Drawing for the job (mm, zero at the part's lowest x, y, z). A direction names the side the tool comes from. Give positions to 0.01 mm unless a question says otherwise; leave off trailing zeros. Write each loop counter-clockwise with the first axis right and the second up, starting at its lowest first coordinate (ties: lowest second). Pieces come first, ordered by that corner, then holes. Notation, with made-up numbers: (-2, 44.25) - (8, 44.25) arc R32 ccw to (8, 79.25) - close; hole circle Ø10 at (3.25, 5.25). An arc over 180 degrees is marked (long way). Write item = value, one per line. Start each with the question number.
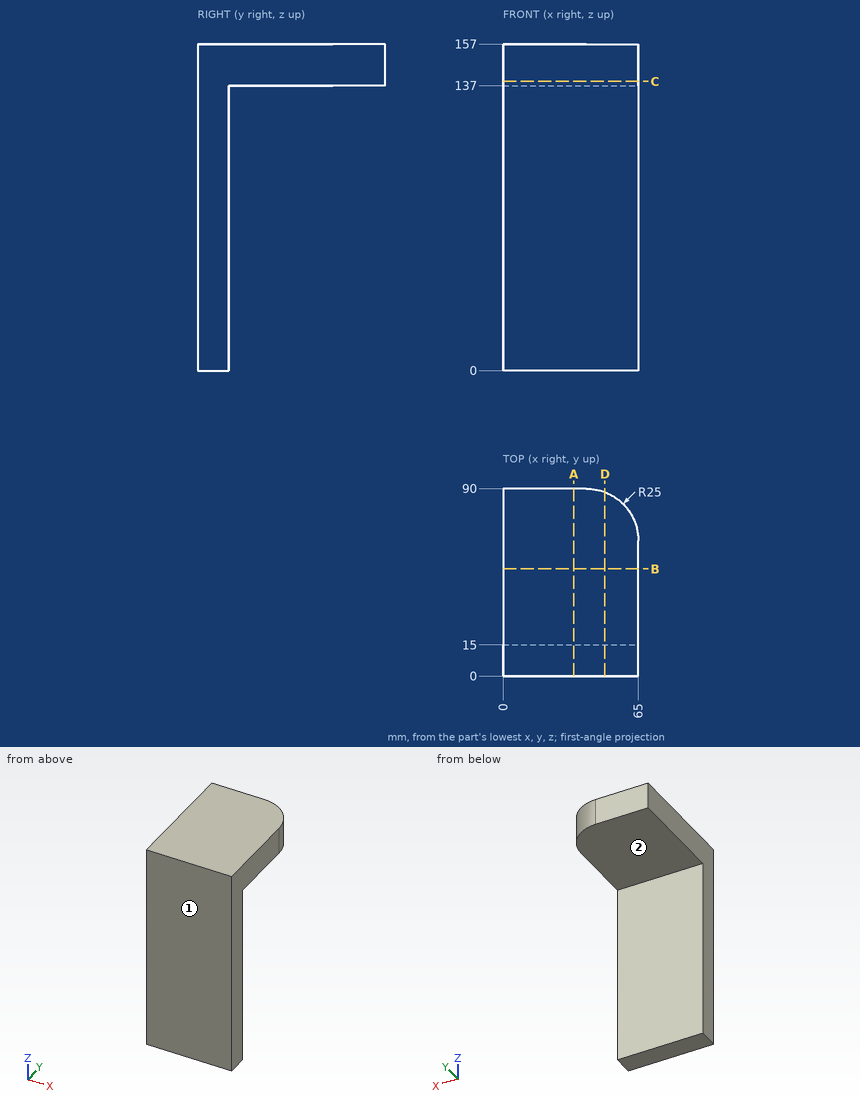
1. Tool access for the marked faces 1 and 2: list every direction of +Z, -Z, +X, -X, +Y, -Y with a clear straight run to the whole face (end or side of a thin tool).
2. Cut at C-C (z = 139). Give the cut face in (x, y).
3. Cut at A-A (x = 34). Give the cut face in (y, z).
4. Cut at B-B (y = 51.5). Give the cut face in (x, z).
5. Cut at D-D (x = 49). Give the cut face in (y, z).
6. Wall check: line 1 along Y through (x, z) = (35, 103.5); line 2 along Z through (x, y) = (42, 33). Give the ranges that are in metal, low to high.
7. Pin check, flat tips, straight feed: pin 1 Ø10 at (x, z) = (49, 66) entering from +Y; pin 2 Ø1 at (x, y) = (43, 54.5) entering from -Z. Stop position of each tip, or through.
Output:
q1.face_1 = +Z, -Z, +X, -X, -Y
q1.face_2 = -Z, +X, -X, +Y
q2.outline = (0, 0) - (65, 0) - (65, 65) arc R25 ccw to (40, 90) - (0, 90) - close
q3.outline = (0, 0) - (15, 0) - (15, 137) - (90, 137) - (90, 157) - (0, 157) - close
q4.outline = (0, 137) - (65, 137) - (65, 157) - (0, 157) - close
q5.outline = (0, 0) - (15, 0) - (15, 137) - (88.32, 137) - (88.32, 157) - (0, 157) - close
q6.line_1 = 0 to 15
q6.line_2 = 137 to 157
q7.pin_1 = 15
q7.pin_2 = 137
